Could you check a few things on this model? Use its own coordinates, in mm. A direction names the side the tool comes from. Round coordinates to 2 decimals unless told otherwise and drop trailing zeros. Loops run counter-clockwise (first coordinate to the right, second up) from the corner with the lowest first, then second, coordinate; pieces in that order, holes last. Notation, with made-up numbers: (63, -17.75) - (102, -17.75) arc R3 ccw to (102, -12.75) - close; hole circle Ø2 at (-37, 66). An arc over 180 degrees is marked (long way). Answer as CSV lines item,"result". Start each with the question number.
1) Suppose I cut it at A-A, the plane y = 8.5. Write out the boundary of the cut face in (x, z), then the cut area to 3 significant figures.
2) Suppose I cut it at C-C, the plane x = -12. Write out the boundary of the cut face in (y, z).
3) Suppose I cut it at B-B, the plane z = 137. Write out the boundary of the cut face in (x, y).
4) I'm going to push flat-ended pins straight in: pin 1 Ø6 at (x, z) = (-0.5, 49) entering from +Y; pin 2 Ø4 at (x, z) = (0, 259) entering from +Y; pin 3 Ø4 at (x, z) = (-2.5, 204) entering from -Y. Where does each tip first touch, or does it pass through?
5) Please list where these lines run through material, in increasing order: line 1 along X through (y, z) = (6, 49.5); line 2 along X through (y, z) = (0.7, 35); line 3 along Y through (x, z) = (20, 232.5).
6) We'd pull the mould along X, two halves only. Please class faces 1 (the face through (22.75, 6, 173)), 2 (the face through (0, 1, 0)), 3 (the face through (0, 1.5, 173)): pulls with the +X half, pulls with the -X half, needs draft (parallel to the pull), parting line crosses it, or undercut.
7) Which directions (+Z, -Z, +X, -X, +Y, -Y) give clear straight access to the entire face, cutting with the end or side of a thin tool? Please do faces 4 (the face through (20.75, 7, 173)), 5 (the face through (0, 0, 173)).
```python
from build123d import *

# Parameters (mm, degrees)
EXTRUDE_1_DEPTH                  = 350
SKETCH_2_R                       = 2.5
CUT_EXTRUDE_1_DEPTH              = 350
PATTERN_LINEAR_1_COUNT           = 2
PATTERN_LINEAR_1_PITCH           = 64
PATTERN_LINEAR_2_COUNT           = 2
PATTERN_LINEAR_2_PITCH           = 160
PATTERN_LINEAR_3_COPY_1_SKETCH_R = 2.5
PATTERN_LINEAR_3_COPY_1_DEPTH    = 350
PATTERN_LINEAR_3_COPY_2_SKETCH_R = 2.5
PATTERN_LINEAR_3_COPY_2_DEPTH    = 350


with BuildPart() as part:
    # 草图1 → 凸台-拉伸1 (new body)
    with BuildSketch(Plane.XY):
        Polygon((-22.75, 0), (22.75, 0), (22.75, 11.5), (20.75, 11.5), (20.75, 1.5), (-20.75, 1.5), (-20.75, 11.5), (-22.75, 11.5), align=None)
    extrude(amount=EXTRUDE_1_DEPTH)

    # 草图2 → 切除-拉伸1 (cut)
    with BuildSketch(Plane.XZ):
        with Locations(Location((0, 35, 0), (0, 0, 270))):
            Circle(SKETCH_2_R)
        with BuildLine():
            Line((2, 52), (2, 48))
            ThreePointArc((2, 48), (0, 46), (-2, 48))
            Line((-2, 48), (-2, 52))
            ThreePointArc((-2, 52), (0, 54), (2, 52))
        make_face()
        with BuildLine():
            Line((-2, 67), (-2, 63))
            ThreePointArc((-2, 63), (0, 61), (2, 63))
            Line((2, 63), (2, 67))
            ThreePointArc((2, 67), (0, 69), (-2, 67))
        make_face()
    cut_extrude_1 = extrude(amount=-CUT_EXTRUDE_1_DEPTH, mode=Mode.SUBTRACT)

    # 阵列(线性)1: 切除-拉伸1 ×2
    with Locations(*[(0, 0, i * PATTERN_LINEAR_1_PITCH) for i in range(1, PATTERN_LINEAR_1_COUNT)]):
        add(cut_extrude_1, mode=Mode.SUBTRACT)

    # 阵列(线性)2: 切除-拉伸1 ×2
    with Locations(*[(0, 0, i * PATTERN_LINEAR_2_PITCH) for i in range(1, PATTERN_LINEAR_2_COUNT)]):
        add(cut_extrude_1, mode=Mode.SUBTRACT)

    # 阵列(线性)3 copy 1 sketch → 阵列(线性)3 copy 1 (cut)
    with BuildSketch(Plane(origin=(0, 0, 224), x_dir=(1, 0, 0), z_dir=(0, -1, 0))):
        with Locations(Location((0, 35, 0), (0, 0, 270))):
            Circle(PATTERN_LINEAR_3_COPY_1_SKETCH_R)
        with BuildLine():
            Line((2, 52), (2, 48))
            ThreePointArc((2, 48), (0, 46), (-2, 48))
            Line((-2, 48), (-2, 52))
            ThreePointArc((-2, 52), (0, 54), (2, 52))
        make_face()
        with BuildLine():
            Line((-2, 67), (-2, 63))
            ThreePointArc((-2, 63), (0, 61), (2, 63))
            Line((2, 63), (2, 67))
            ThreePointArc((2, 67), (0, 69), (-2, 67))
        make_face()
    extrude(amount=-PATTERN_LINEAR_3_COPY_1_DEPTH, mode=Mode.SUBTRACT)

    # 阵列(线性)3 copy 2 sketch → 阵列(线性)3 copy 2 (cut)
    with BuildSketch(Plane(origin=(0, 0, 160), x_dir=(1, 0, 0), z_dir=(0, -1, 0))):
        with Locations(Location((0, 35, 0), (0, 0, 270))):
            Circle(PATTERN_LINEAR_3_COPY_2_SKETCH_R)
        with BuildLine():
            Line((2, 52), (2, 48))
            ThreePointArc((2, 48), (0, 46), (-2, 48))
            Line((-2, 48), (-2, 52))
            ThreePointArc((-2, 52), (0, 54), (2, 52))
        make_face()
        with BuildLine():
            Line((-2, 67), (-2, 63))
            ThreePointArc((-2, 63), (0, 61), (2, 63))
            Line((2, 63), (2, 67))
            ThreePointArc((2, 67), (0, 69), (-2, 67))
        make_face()
    extrude(amount=-PATTERN_LINEAR_3_COPY_2_DEPTH, mode=Mode.SUBTRACT)


solid = part.part
```
Filled sheet:
1,outline,"(-22.75, 0) - (-20.75, 0) - (-20.75, 350) - (-22.75, 350) - close; (20.75, 0) - (22.75, 0) - (22.75, 350) - (20.75, 350) - close"
1,area,"1,400 mm²"
2,outline,"(0, 0) - (1.5, 0) - (1.5, 350) - (0, 350) - close"
3,outline,"(-22.75, 0) - (22.75, 0) - (22.75, 11.5) - (20.75, 11.5) - (20.75, 1.5) - (-20.75, 1.5) - (-20.75, 11.5) - (-22.75, 11.5) - close"
4,pin 1,"y = 1.5"
4,pin 2,"through"
4,pin 3,"y = 0"
5,line 1,"-22.75 to -20.75, 20.75 to 22.75"
5,line 2,"-22.75 to -2.5, 2.5 to 22.75"
5,line 3,"0 to 1.5"
6,face 1,"pulls with the +X half"
6,face 2,"needs draft"
6,face 3,"undercut"
7,face 4,"+Z, -Z, +Y"
7,face 5,"+Z, -Z, +X, -X, -Y"
